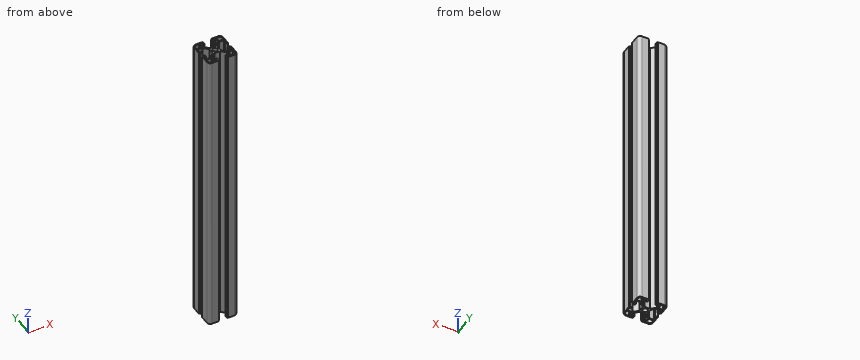
from build123d import *

# Parameters (mm, degrees)
BOSS_EXTRUDE1_DEPTH  = 410
MIRROR3_COPY_1_DEPTH = 410
MIRROR3_COPY_2_DEPTH = 410


with BuildPart() as part:
    # Sketch1 → Boss-Extrude1 (new body)
    with BuildSketch(Plane.XY):
        with BuildLine():
            Line((3.4, 0), (5.5, 0))
            Line((5.5, 0), (5.5, 4))
            Line((5.5, 4), (11.69, 10.19))
            Line((11.69, 10.19), (18.2, 10.19))
            Line((18.2, 10.19), (18.2, 5.265595036))
            Line((18.2, 5.265595036), (15.5, 5.265595036))
            Line((15.5, 5.265595036), (15.5, 2.965595036))
            Line((15.5, 2.965595036), (19, 2.965595036))
            Line((19, 2.965595036), (19, 3.965595036))
            Line((19, 3.965595036), (20, 3.965595036))
            Line((20, 3.965595036), (20, 15.5))
            ThreePointArc((20, 15.5), (18.681980515, 18.681980515), (15.5, 20))
            Line((15.5, 20), (6.385304712, 20))
            Line((6.385304712, 20), (6.385304712, 19))
            Line((6.385304712, 19), (5.385304712, 19))
            Line((5.385304712, 19), (5.385304712, 15.5))
            Line((5.385304712, 15.5), (7.685304712, 15.5))
            Line((7.685304712, 15.5), (7.685304712, 18.2))
            Line((7.685304712, 18.2), (10.19, 18.2))
            Line((10.19, 18.2), (10.19, 11.69))
            Line((10.19, 11.69), (4, 5.5))
            Line((4, 5.5), (0, 5.5))
            Line((0, 5.5), (0, 3.4))
            ThreePointArc((0, 3.4), (2.404163056, 2.404163056), (3.4, 0))
        make_face()
        with BuildLine():
            Line((18.5, 11.69), (18.5, 15.5))
            ThreePointArc((18.5, 15.5), (17.621320344, 17.621320344), (15.5, 18.5))
            Line((15.5, 18.5), (11.69, 18.5))
            Line((11.69, 18.5), (11.69, 11.69))
            Line((11.69, 11.69), (18.5, 11.69))
        make_face(mode=Mode.SUBTRACT)
    boss_extrude1 = extrude(amount=BOSS_EXTRUDE1_DEPTH)

    # Mirror1: Boss-Extrude1 across plane
    add(boss_extrude1.mirror(Plane.ZX))

    # Mirror2: Boss-Extrude1 across plane
    add(boss_extrude1.mirror(Plane(origin=(0, 0, 0), x_dir=(0, 0, 1), z_dir=(1, 0, 0))))

    # Mirror3 copy 1 sketch → Mirror3 copy 1 (add)
    with BuildSketch(Plane(origin=(0, 0, 0), x_dir=(-1, 0, 0), z_dir=(0, 0, 1))):
        with BuildLine():
            Line((3.4, 0), (5.5, 0))
            Line((5.5, 0), (5.5, 4))
            Line((5.5, 4), (11.69, 10.19))
            Line((11.69, 10.19), (18.2, 10.19))
            Line((18.2, 10.19), (18.2, 5.265595036))
            Line((18.2, 5.265595036), (15.5, 5.265595036))
            Line((15.5, 5.265595036), (15.5, 2.965595036))
            Line((15.5, 2.965595036), (19, 2.965595036))
            Line((19, 2.965595036), (19, 3.965595036))
            Line((19, 3.965595036), (20, 3.965595036))
            Line((20, 3.965595036), (20, 15.5))
            ThreePointArc((20, 15.5), (18.681980515, 18.681980515), (15.5, 20))
            Line((15.5, 20), (6.385304712, 20))
            Line((6.385304712, 20), (6.385304712, 19))
            Line((6.385304712, 19), (5.385304712, 19))
            Line((5.385304712, 19), (5.385304712, 15.5))
            Line((5.385304712, 15.5), (7.685304712, 15.5))
            Line((7.685304712, 15.5), (7.685304712, 18.2))
            Line((7.685304712, 18.2), (10.19, 18.2))
            Line((10.19, 18.2), (10.19, 11.69))
            Line((10.19, 11.69), (4, 5.5))
            Line((4, 5.5), (0, 5.5))
            Line((0, 5.5), (0, 3.4))
            ThreePointArc((0, 3.4), (2.404163056, 2.404163056), (3.4, 0))
        make_face()
        with BuildLine():
            Line((18.5, 11.69), (18.5, 15.5))
            ThreePointArc((18.5, 15.5), (17.621320344, 17.621320344), (15.5, 18.5))
            Line((15.5, 18.5), (11.69, 18.5))
            Line((11.69, 18.5), (11.69, 11.69))
            Line((11.69, 11.69), (18.5, 11.69))
        make_face(mode=Mode.SUBTRACT)
    extrude(amount=MIRROR3_COPY_1_DEPTH)

    # Mirror3 copy 2 sketch → Mirror3 copy 2 (add)
    with BuildSketch(Plane.XY):
        with BuildLine():
            Line((3.4, 0), (5.5, 0))
            Line((5.5, 0), (5.5, -4))
            Line((5.5, -4), (11.69, -10.19))
            Line((11.69, -10.19), (18.2, -10.19))
            Line((18.2, -10.19), (18.2, -5.265595036))
            Line((18.2, -5.265595036), (15.5, -5.265595036))
            Line((15.5, -5.265595036), (15.5, -2.965595036))
            Line((15.5, -2.965595036), (19, -2.965595036))
            Line((19, -2.965595036), (19, -3.965595036))
            Line((19, -3.965595036), (20, -3.965595036))
            Line((20, -3.965595036), (20, -15.5))
            ThreePointArc((20, -15.5), (18.681980515, -18.681980515), (15.5, -20))
            Line((15.5, -20), (6.385304712, -20))
            Line((6.385304712, -20), (6.385304712, -19))
            Line((6.385304712, -19), (5.385304712, -19))
            Line((5.385304712, -19), (5.385304712, -15.5))
            Line((5.385304712, -15.5), (7.685304712, -15.5))
            Line((7.685304712, -15.5), (7.685304712, -18.2))
            Line((7.685304712, -18.2), (10.19, -18.2))
            Line((10.19, -18.2), (10.19, -11.69))
            Line((10.19, -11.69), (4, -5.5))
            Line((4, -5.5), (0, -5.5))
            Line((0, -5.5), (0, -3.4))
            ThreePointArc((0, -3.4), (2.404163056, -2.404163056), (3.4, 0))
        make_face()
        with BuildLine():
            Line((18.5, -11.69), (18.5, -15.5))
            ThreePointArc((18.5, -15.5), (17.621320344, -17.621320344), (15.5, -18.5))
            Line((15.5, -18.5), (11.69, -18.5))
            Line((11.69, -18.5), (11.69, -11.69))
            Line((11.69, -11.69), (18.5, -11.69))
        make_face(mode=Mode.SUBTRACT)
    extrude(amount=MIRROR3_COPY_2_DEPTH)


solid = part.part
Input: part model. Units: mm. Frame: model coordinates. Coordinates: 2 decimals unless noted, no trailing zeros. One line per item, written item: value.
(1) Cut plane A-A (z = 130). Give the number of separate pieces and of enclosed holes in the cut face, then the cut area to 3 significant figures.
Answer below:
separate pieces: 1
enclosed holes: 5
area: 468 mm2
(2) Ray query, line 1 along Y through (x, z) = (-13.5, 258); line 2 along X through (y, z) = (16, 264). Return the intervals inside material, ascending.
Answer below:
line 1: y = -20 to -18.5, -11.69 to -10.19, 10.19 to 11.69, 18.5 to 20
line 2: x = -19.97 to -18.46, -11.69 to -10.19, -7.69 to -5.39, 5.39 to 7.69, 10.19 to 11.69, 18.46 to 19.97
(3) Pin query (flat end, axial travel): pin 1 Ø1.1 at (x, z) = (19.5, 304.5) entering from +Y; pin 2 Ø1.3 at (x, z) = (-16.5, 299.5) entering from +Y; pin 3 Ø1.1 at (y, z) = (-19.5, 242.5) entering from +X. Return the tip coordinate at first contact, or that it passes through.
Answer below:
pin 1: stops at y = 18.39
pin 2: stops at y = 19.99
pin 3: stops at x = 18.39
